Input: part model. Units: mm. Frame: model coordinates. Face numbers are marked on the shaded views. A direction names the side the tool comes from. Coordinates: 2 decimals unless noted, no trailing zeros. Order: outer loops, then holes, each group sorted by start corner. A loop starts at its lowest first (then second) coordinate and runs counter-clockwise, first axis right, second up. Notation, with made-up numbers: (-3.5, 80.25) -> (34.5, 80.25) arc R24 cw to (34.5, 101.25) -> close; hole circle Ø8 at (-35, -23). An arc over 180 degrees is marked (long way). One line per question, with ' | ' between items.
```python
from build123d import *

# Parameters (mm, degrees)
BOSS_EXTRU_1_DEPTH      = 6
BOSS_EXTRU_2_DEPTH      = 20.3
BOSS_EXTRU_3_DEPTH      = 6
BOSS_EXTRU_4_DEPTH      = 30
ESQUISSE5_R             = 1.5
ENL_V_MAT_EXTRU_1_DEPTH = 30
ESQUISSE6_R             = 1.5
ENL_V_MAT_EXTRU_2_DEPTH = 30
ESQUISSE7_R             = 2
ENL_V_MAT_EXTRU_3_DEPTH = 30
CHANFREIN1_SIZE         = 2


with BuildPart() as part:
    # Esquisse1 → Boss.-Extru.1 (new body)
    with BuildSketch(Plane(origin=(0, 0, 0), x_dir=(1, 0, 0), z_dir=(0, 1, 0))):
        Polygon((22.839549032, 45.679098065), (100, 8.485281374), (22.839549032, 8.485281374), align=None)
        Polygon((22.839549032, 45.679098065), (0, 45.679098065), (0, 0), (100, 0), (100, 8.485281374), (22.839549032, 8.485281374), align=None)
    extrude(amount=BOSS_EXTRU_1_DEPTH)

    # Esquisse2 → Boss.-Extru.2 (add)
    with BuildSketch(Plane(origin=(0, 6, 0), x_dir=(1, 0, 0), z_dir=(0, 1, 0))):
        Polygon((22.839549032, 45.679098065), (10.15, 45.679098065), (10.15, 6), (0, 6), (0, 0), (100, 0), (100, 8.485281374), (22.839549032, 8.485281374), align=None)
    extrude(amount=BOSS_EXTRU_2_DEPTH)

    # Esquisse3 → Boss.-Extru.3 (add)
    with BuildSketch(Plane(origin=(0, 26.3, 0), x_dir=(1, 0, 0), z_dir=(0, 1, 0))):
        Polygon((22.839549032, 45.679098065), (0, 45.679098065), (0, 0), (100, 0), (100, 8.485281374), (22.839549032, 8.485281374), align=None)
    extrude(amount=BOSS_EXTRU_3_DEPTH)

    # Esquisse4 → Boss.-Extru.4 (add)
    with BuildSketch(Plane(origin=(0, 32.3, 0), x_dir=(1, 0, 0), z_dir=(0, 1, 0))):
        Polygon((0, 0), (22.839549032, 22.839548119), (0, 45.679098065), (0, 37.193816521), (14.354267489, 22.839548459), (0, 8.485281544), align=None)
    extrude(amount=BOSS_EXTRU_4_DEPTH)

    # Esquisse5 → Enlèv. mat.-Extru.1 (cut)
    with BuildSketch(Plane(origin=(22.839549032, 0, -22.839548119), x_dir=(-0.7071067670543795, 0, -0.7071067953187153), z_dir=(0.7071067953187153, 0, -0.7071067670543795))):
        with Locations((16.150000323, 52.3)):
            Circle(ESQUISSE5_R)
    extrude(amount=-ENL_V_MAT_EXTRU_1_DEPTH, mode=Mode.SUBTRACT)

    # Esquisse6 → Enlèv. mat.-Extru.2 (cut)
    with BuildSketch(Plane(origin=(22.839549032, 0, 0), x_dir=(0, 0, -1), z_dir=(1, 0, 0))):
        with Locations((30.679098065, 19.15)):
            Circle(ESQUISSE6_R)
    extrude(amount=-ENL_V_MAT_EXTRU_2_DEPTH, mode=Mode.SUBTRACT)

    # Esquisse7 → Enlèv. mat.-Extru.3 (cut)
    with BuildSketch(Plane(origin=(0, 0, -8.485281374), x_dir=(-1, 0, 0), z_dir=(0, 0, -1))):
        with Locations((-41.419774516, 19.15)):
            Circle(ESQUISSE7_R)
        with Locations((-81.419774516, 19.15)):
            Circle(ESQUISSE7_R)
    extrude(amount=-ENL_V_MAT_EXTRU_3_DEPTH, mode=Mode.SUBTRACT)

    # Chanfrein1
    chanfrein1_edges = [part.edges().sort_by_distance(p)[0] for p in [
        (12.480434667, 52.3, -33.198662899),
        (22.839549032, 19.15, -29.179098065),
        (43.419774516, 19.15, -8.485281374),
        (83.419774516, 19.15, -8.485281374),
    ]]
    chamfer(chanfrein1_edges, length=CHANFREIN1_SIZE)

    # Symétrie1: part across plane


with BuildPart() as part_1:
    add(part.part)
    add(part.part.mirror(Plane(origin=(0, 6, 0), x_dir=(0, 0, 1), z_dir=(1, 0, 0))))


solid = part_1.part
```
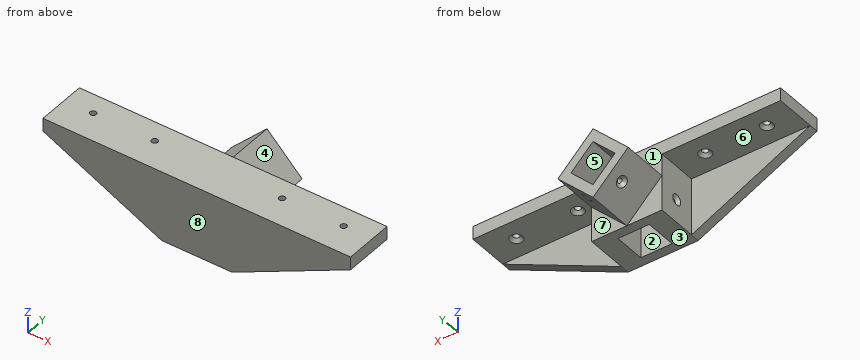
1. Cut plane D-D, the plane z = -21. Return loops of the section in (x, y), and give its area (3 significant figures).
Recorded:
outline: (-74.04, 0) -> (74.04, 0) -> (74.04, 6) -> (22.84, 6) -> (22.84, 32.3) -> (21, 32.3) -> (21, 62.3) -> (12.51, 62.3) -> (12.51, 32.3) -> (-12.51, 32.3) -> (-12.51, 62.3) -> (-21, 62.3) -> (-21, 32.3) -> (-22.84, 32.3) -> (-22.84, 6) -> (-74.04, 6) -> close; hole (-10.15, 6) -> (10.15, 6) -> (10.15, 26.3) -> (-10.15, 26.3) -> close | area: 2,190 mm^2
2. Ray query, line 1 (X direction, y = 14.5, z = -28); line 2 (Z direction, x = 13, y = 19); line 3 (Y direction, x = -1, z = -16.5). Return the intervals inside material, ascending. Write a range as [from, to].
Recorded:
line 1: x = [-22.84, -10.15], [10.15, 22.84] | line 2: z = [-45.68, -32.17], [-29.19, 0] | line 3: y = [0, 6], [26.3, 32.3]
3. Pin query (flat end, axial travel): pin 1 Ø21 at (x, y) = (68.5, 25) entering from -Z; pin 2 Ø10 at (x, z) = (65, -25) entering from +Y; pin 3 Ø3.5 at (x, y) = (81.42, 19.15) entering from -Z; pin 4 Ø6.5 at (x, y) = (41.42, 19.15) entering from -Z. Return the tip coordinate at first contact, or that it passes through.
Recorded:
pin 1: stops at z = -8.49 | pin 2: stops at y = 6 | pin 3: passes through | pin 4: stops at z = -7.74
4. Cut plane B-B, the plane y = 12.5. Return loops of the section in (x, z), and give its area (3 significant figures).
Recorded:
outline: (-100, -8.49) -> (-22.84, -8.49) -> (-22.84, -45.68) -> (-10.15, -45.68) -> (-10.15, -6) -> (10.15, -6) -> (10.15, -45.68) -> (22.84, -45.68) -> (22.84, -8.49) -> (100, -8.49) -> (100, 0) -> (-100, 0) -> close | area: 2,590 mm^2
5. Cut plane C-C, the plane x = 60. Return loops of the section in (y, z), and give its area (3 significant figures).
Recorded:
outline: (0, -27.77) -> (6, -27.77) -> (6, -8.49) -> (32.3, -8.49) -> (32.3, 0) -> (0, 0) -> close | area: 390 mm^2
6. Mould query, pull axis Y, two halves, no side actions, for the marked faces 1, 2 and 3. Classes: released by +Y, released by -Y, zero draft, split by the parting line, or undercut.
Recorded:
face 1: released by +Y | face 2: undercut | face 3: zero draft
7. Access query for the marked faces 4, 5, 6, 7 and 8. Directions: +Z, -Z, +X, -X, +Y, -Y. A direction counts if a zero-diameter tool reaches every point of the face in a straight line with its end or side. Return the directions, or none.
Recorded:
face 4: +Z, +X, +Y | face 5: +Y | face 6: -Z, -X, +Y | face 7: -Z, +X, +Y | face 8: +Z, -Z, +X, -X, -Y
8. Cut plane A-A, the plane z = -41.5. Return loops of the section in (x, y).
Recorded:
outline: (-31.51, 0) -> (31.51, 0) -> (31.51, 6) -> (22.84, 6) -> (22.84, 32.3) -> (4.18, 32.3) -> (4.18, 62.3) -> (-4.18, 62.3) -> (-4.18, 32.3) -> (-22.84, 32.3) -> (-22.84, 6) -> (-31.51, 6) -> close; hole (-10.15, 6) -> (10.15, 6) -> (10.15, 26.3) -> (-10.15, 26.3) -> close
